```python
from build123d import *

# Parameters (mm, degrees)
SKETCH1_R           = 11.5
SKETCH1_R_2         = 1.5
BOSS_EXTRUDE1_DEPTH = 5


with BuildPart() as part:
    # Sketch1 → Boss-Extrude1 (new body)
    with BuildSketch(Plane(origin=(0, 0, 0), x_dir=(1, 0, 0), z_dir=(0, 1, 0))):
        Polygon((-39.35, -15), (-37.35, -15), (-37.35, -19), (-27.35, -19), (-27.35, -15), (-21.15, -15), (-21.15, -21.15), (21.15, -21.15), (21.15, -15), (27.35, -15), (27.35, -19), (37.35, -19), (37.35, -15), (39.35, -15), (39.35, 15), (37.35, 15), (37.35, 19), (27.35, 19), (27.35, 15), (21.15, 15), (21.15, 21.15), (-21.15, 21.15), (-21.15, 15), (-27.35, 15), (-27.35, 19), (-37.35, 19), (-37.35, 15), (-39.35, 15), align=None)
        Circle(SKETCH1_R, mode=Mode.SUBTRACT)
        with Locations((15.5, 15.5)):
            Circle(SKETCH1_R_2, mode=Mode.SUBTRACT)
        with Locations((15.5, -15.5)):
            Circle(SKETCH1_R_2, mode=Mode.SUBTRACT)
        with Locations((-15.5, -15.5)):
            Circle(SKETCH1_R_2, mode=Mode.SUBTRACT)
        with Locations((-15.5, 15.5)):
            Circle(SKETCH1_R_2, mode=Mode.SUBTRACT)
    extrude(amount=BOSS_EXTRUDE1_DEPTH)


solid = part.part
```
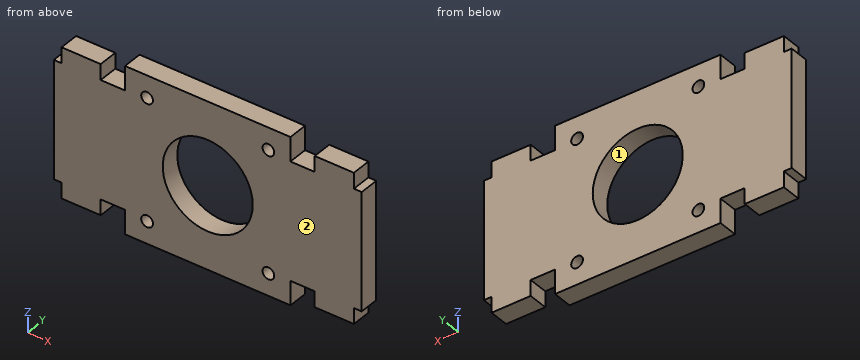
Could you check a few things on this model? Use its own coordinates, in mm. Face numbers are marked on the shaded views. Give positions to 0.01 mm unless a question says otherwise; leave off trailing zeros. Order: outer loops, then holes, each group sorted by start corner. A loop starts at its lowest first (then second) coordinate and runs counter-clockwise, first axis right, second up.
Q1. I'm going to push flat-ended pins straight in: P1, Ø2, axis at x = -38.5, y = 3.5, coming from the +Z side; P2, Ø0.6, axis at x = 38.5, y = 2, coming from the -Z side; P3, Ø2, axis at y = 3, z = -17.5, coming from the -X side. Where does each tip first touch, or does it pass through?
Q2. Suppose I cut it at D-D, the plane z = -7.5. Write out the boundary of the cut face in (x, y), and give its area (3 significant figures).
Q3. We'd pull the mould along X, two halves only. Please class the marked faces 1 and 2: +X half, -X half, draft (parallel to the pull), parting line (faces both ways), or undercut.
Q4. If I drill on line 1 along Z through (x, y) = (-15.5, 1.8); line 2 along X through (y, z) = (1.65, 15.5); line 3 along X through (y, z) = (2.85, 0), over which ranges is the centre line in solid material (lowest first)?
Q5. Suppose I cut it at B-B, the plane x = -15.5. Write out the boundary of the cut face in (y, z), and give its area (4 significant figures).
Q6. Suppose I cut it at A-A, the plane z = 0. Write out the boundary of the cut face in (x, y), and give its area (4 significant figures).
Q7. Suppose I cut it at C-C, the plane y = 1.55. Count the separate pieces of the cut face and the enclosed holes in it, and give its area (3 significant figures).
Solution:
1. P1: stops at z = 15
1. P2: stops at z = -15
1. P3: stops at x = -37.35
2. outline: (-39.35, 0) - (-8.72, 0) - (-8.72, 5) - (-39.35, 5) - close; (8.72, 0) - (39.35, 0) - (39.35, 5) - (8.72, 5) - close
2. area: 306 mm2
3. face 1: undercut
3. face 2: draft
4. line 1: z = -21.15 to -17, -14 to 14, 17 to 21.15
4. line 2: x = -37.35 to -27.35, -21.15 to -17, -14 to 14, 17 to 21.15, 27.35 to 37.35
4. line 3: x = -39.35 to -11.5, 11.5 to 39.35
5. outline: (0, -21.15) - (5, -21.15) - (5, -17) - (0, -17) - close; (0, -14) - (5, -14) - (5, 14) - (0, 14) - close; (0, 17) - (5, 17) - (5, 21.15) - (0, 21.15) - close
5. area: 181.5 mm2
6. outline: (-39.35, 0) - (-11.5, 0) - (-11.5, 5) - (-39.35, 5) - close; (11.5, 0) - (39.35, 0) - (39.35, 5) - (11.5, 5) - close
6. area: 278.5 mm2
7. separate pieces: 1
7. enclosed holes: 5
7. area: 2,600 mm2
